```python
from build123d import *

# Parameters (mm, degrees)
SALIENTE_EXTRUIR1_DEPTH  = 0.9
CROQUIS2_W               = 1.87835833
CROQUIS2_H               = 5
SALIENTE_EXTRUIR2_DEPTH  = 0.3
CROQUIS3_W               = 4
CROQUIS3_H               = 5
SALIENTE_EXTRUIR4_DEPTH  = 1.7
CROQUIS4_W               = 4
CROQUIS4_H               = 5
SALIENTE_EXTRUIR5_DEPTH  = 1.7
CROQUIS5_W               = 1
CROQUIS5_H               = 15.8
SALIENTE_EXTRUIR6_DEPTH  = 10
SALIENTE_EXTRUIR8_START  = -3.14
SALIENTE_EXTRUIR8_DEPTH  = 2.16
SALIENTE_EXTRUIR9_START  = -3.14
SALIENTE_EXTRUIR9_DEPTH  = 2.16
SALIENTE_EXTRUIR10_DEPTH = 1
SALIENTE_EXTRUIR11_DEPTH = 1
CROQUIS14_W              = 1.5
CROQUIS14_H              = 7.3
CORTAR_EXTRUIR1_DEPTH    = 4.7
CROQUIS16_W              = 2
CROQUIS16_H              = 9.52
CORTAR_EXTRUIR2_DEPTH    = 4.7


with BuildPart() as part:
    # Croquis1 → Saliente-Extruir1 (new body)
    with BuildSketch(Plane(origin=(0, 0, 0), x_dir=(1, 0, 0), z_dir=(0, 1, 0))):
        Polygon((-13.741322015, -0.507016954), (-13.741322015, -12.507016954), (40.258677985, -12.507016954), (40.258677985, 15.992983046), (-13.741322015, 15.992983046), (-13.741322015, 3.992983046), (-15.191322015, 3.992983046), (-15.191322015, -0.507016954), align=None)
    extrude(amount=SALIENTE_EXTRUIR1_DEPTH)

    # Croquis2 → Saliente-Extruir2 (add)
    with BuildSketch(Plane(origin=(0, 0.9, 0), x_dir=(1, 0, 0), z_dir=(0, 1, 0))):
        with Locations((39.31949882, -4.007016954)):
            Rectangle(CROQUIS2_W, CROQUIS2_H)
        with Locations((39.31949882, 7.492983046)):
            Rectangle(CROQUIS2_W, CROQUIS2_H)
    extrude(amount=SALIENTE_EXTRUIR2_DEPTH)

    # Croquis3 → Saliente-Extruir4 (add)
    with BuildSketch(Plane(origin=(0, 1.2, 0), x_dir=(1, 0, 0), z_dir=(0, 1, 0))):
        with Locations((40.380319655, -4.007016954)):
            Rectangle(CROQUIS3_W, CROQUIS3_H)
    extrude(amount=SALIENTE_EXTRUIR4_DEPTH)

    # Croquis4 → Saliente-Extruir5 (add)
    with BuildSketch(Plane(origin=(0, 1.2, 0), x_dir=(1, 0, 0), z_dir=(0, 1, 0))):
        with Locations((40.380319655, 7.492983046)):
            Rectangle(CROQUIS4_W, CROQUIS4_H)
    extrude(amount=SALIENTE_EXTRUIR5_DEPTH)

    # Croquis5 → Saliente-Extruir6 (add)
    with BuildSketch(Plane(origin=(0, 0.9, 0), x_dir=(1, 0, 0), z_dir=(0, 1, 0))):
        with Locations((-13.241322015, 1.742983046)):
            Rectangle(CROQUIS5_W, CROQUIS5_H)
    extrude(amount=SALIENTE_EXTRUIR6_DEPTH)

    # Croquis6 → Saliente-Extruir8 (add)
    with BuildSketch(Plane(origin=(0, 0, -9.642983046), x_dir=(-1, 0, 0), z_dir=(0, 0, -1)).offset(SALIENTE_EXTRUIR8_START)):
        Polygon((13.741322015, 2.5), (13.741322015, 5.5), (15.741322015, 2.5), align=None)
    extrude(amount=-SALIENTE_EXTRUIR8_DEPTH)

    # Croquis9 → Saliente-Extruir9 (add)
    with BuildSketch(Plane.XY.offset(6.157016954).offset(SALIENTE_EXTRUIR9_START)):
        Polygon((-15.741322015, 2.5), (-13.741322015, 5.5), (-13.741322015, 2.5), align=None)
    extrude(amount=-SALIENTE_EXTRUIR9_DEPTH)

    # Croquis12 → Saliente-Extruir10 (add)
    with BuildSketch(Plane(origin=(0, 0, -9.642983046), x_dir=(-1, 0, 0), z_dir=(0, 0, -1))):
        Polygon((12.741322015, 0.9), (9.741322015, 0.9), (12.741322015, 6.9), align=None)
    extrude(amount=-SALIENTE_EXTRUIR10_DEPTH)

    # Croquis13 → Saliente-Extruir11 (add)
    with BuildSketch(Plane.XY.offset(6.157016954)):
        Polygon((-12.741322015, 0.9), (-9.741322015, 0.9), (-12.741322015, 6.9), align=None)
    extrude(amount=-SALIENTE_EXTRUIR11_DEPTH)

    # Croquis14 → Cortar-Extruir1 (cut)
    with BuildSketch(Plane.ZY.offset(13.741322015)):
        with Locations((3.767016954, 3.65)):
            Rectangle(CROQUIS14_W, CROQUIS14_H)
        with Locations((-7.252983046, 3.65)):
            Rectangle(CROQUIS14_W, CROQUIS14_H)
    extrude(amount=-CORTAR_EXTRUIR1_DEPTH, mode=Mode.SUBTRACT)

    # Croquis16 → Cortar-Extruir2 (cut)
    with BuildSketch(Plane(origin=(0, 0.9, 0), x_dir=(1, 0, 0), z_dir=(0, 1, 0))):
        with Locations((-10.041322015, 1.742983046)):
            Rectangle(CROQUIS16_W, CROQUIS16_H)
    extrude(amount=-CORTAR_EXTRUIR2_DEPTH, mode=Mode.SUBTRACT)


solid = part.part
```
Geometry check sheet. Reference: the model listing, model coordinates, mm. A direction names the side the tool comes from. Coordinates: 2 decimals unless noted, no trailing zeros. Loops run counter-clockwise (first coordinate to the right, second up) from the corner with the lowest first, then second, coordinate; pieces in that order, holes last. Notation, with made-up numbers: (7.5, 18) -> (49.5, 18) arc R12 cw to (49.5, 23) -> close; hole circle Ø6 at (13, -34.75). An arc over 180 degrees is marked (long way). Put each result on its own line as item: value.
1) Cross-section at B-B on x = -5.5. Record the boundary of the cut face in (y, z), plus the area to 4 significant figures.
Result set:
outline: (0, -15.99) -> (0.9, -15.99) -> (0.9, 12.51) -> (0, 12.51) -> close
area: 25.65 mm^2
2) Gauge pin test, flat ends, axial feed: pin 1 Ø0.6 at (x, z) = (41.5, 4) entering from -Y; pin 2 Ø4 at (x, z) = (22.5, -7) entering from +Y; pin 3 Ø4.5 at (x, z) = (40.5, -8) entering from +Y; pin 4 Ø5 at (x, y) = (-9.5, 6.5) entering from +Z. Record the tip position at first contact, or that the pin passes through.
Result set:
pin 1: stops at y = 1.2
pin 2: stops at y = 0.9
pin 3: stops at y = 2.9
pin 4: passes through
3) Thickness scan on line 1 (Z direction, x = -10, y = 0.5); line 2 (Y direction, x = 38.5, z = 6); line 3 (Y direction, x = 3.5, z = 1.25). Record the ranges inside material, lowest first.
Result set:
line 1: z = -15.99 to -8, 4.52 to 12.51
line 2: y = 0 to 2.9
line 3: y = 0 to 0.9
4) Cross-section at C-C on y = 10. Record the boundary of the cut face in (x, z), plus the area to 3 significant figures.
Result set:
outline: (-13.74, -9.64) -> (-12.74, -9.64) -> (-12.74, 6.16) -> (-13.74, 6.16) -> close
area: 15.8 mm^2
5) Release check for a two-part mould opening along Z. For faces 1 (the flat face through (38.38, 2, 4)), 2 (the flat face through (40, 2, -4.993)), 3 (the flat face through (-13, 5, 6.157)) record: released by +Z, released by -Z, zero draft, split by the parting line, or undercut.
Result set:
face 1: zero draft
face 2: undercut
face 3: released by +Z
6) Cross-section at A-A on y = 3.5. Record the boundary of the cut face in (x, z).
Result set:
outline: (-15.07, -6.5) -> (-12.74, -6.5) -> (-12.74, 3.02) -> (-15.07, 3.02) -> (-15.07, 0.86) -> (-13.74, 0.86) -> (-13.74, -4.34) -> (-15.07, -4.34) -> close; (-13.74, -9.64) -> (-11.04, -9.64) -> (-11.04, -8.64) -> (-12.74, -8.64) -> (-12.74, -8) -> (-13.74, -8) -> close; (-13.74, 4.52) -> (-12.74, 4.52) -> (-12.74, 5.16) -> (-11.04, 5.16) -> (-11.04, 6.16) -> (-13.74, 6.16) -> close
7) Tool access check on faces 4 (the flat face through (-13, 3, -8.003)), 5 (the flat face through (40, 2, 1.507)), 6 (the flat face through (-12, 3, -8.643)), 7 (the flat face through (40.259, 0.5, -1.5)), 8 (the flat face through (40, 2.9, -8)). Record the directions out of +Z, -Z, +X, -X, +Y, -Y that give a thin tool (end or side, any length) a straight path to the whole face; none if there is none.
Result set:
face 4: -X, -Y
face 5: +X, +Y
face 6: +Y
face 7: +Z, -Z, +X, -Y
face 8: +Z, -Z, +X, +Y
